```python
from build123d import *

# Parameters (mm, degrees)
SKETCH2_W               = 20
SKETCH2_H               = 10
BOSS_EXTRUDE1_DEPTH     = 132
SKETCH6_W               = 10
SKETCH6_H               = 3
BOSS_EXTRUDE2_DEPTH     = 10
FILLET2_R               = 10
CUT_EXTRUDE5_DEPTH      = 131.636901372
CUT_EXTRUDE5_DEPTH_BACK = 131.636901372
SKETCH19_R              = 1.5
SKETCH19_5_R            = 2.7
SKETCH19_5_R_2          = 1.5
CUT_EXTRUDE7_DEPTH      = 131.636901376
FILLET1_R               = 1
FILLET3_R               = 10
CUT_EXTRUDE8_DEPTH      = 131.636901391
CUT_EXTRUDE8_DEPTH_BACK = 131.636901391
SKETCH20_R              = 1.5
SKETCH20_3_R            = 2.7
SKETCH20_3_R_2          = 1.5
CUT_EXTRUDE9_DEPTH      = 131.636901391
SKETCH21_R              = 2.5
CUT_EXTRUDE10_DEPTH     = 10
FILLET4_R               = 15


# Some blends are built 0.0001 mm under size
with BuildPart() as part:
    # Sketch2 → Boss-Extrude1 (new body)
    with BuildSketch(Plane(origin=(0, 0, 0), x_dir=(1, 0, 0), z_dir=(0, 1, 0))):
        Rectangle(SKETCH2_W, SKETCH2_H)
    extrude(amount=BOSS_EXTRUDE1_DEPTH)

    # Sketch6 → Boss-Extrude2 (add)
    with BuildSketch(Plane(origin=(10, 0, 0), x_dir=(0, 0, -1), z_dir=(1, 0, 0))):
        with Locations((0, 1.5)):
            Rectangle(SKETCH6_W, SKETCH6_H)
    boss_extrude2 = extrude(amount=BOSS_EXTRUDE2_DEPTH)

    # Fillet2
    fillet2_edges = [part.edges().sort_by_distance(p)[0] for p in [
        (10, 3, 0),
    ]]
    fillet(fillet2_edges, radius=FILLET2_R - 0.0001)  # a hair under: the kernel refuses the full size

    # Sketch19 → Cut-Extrude5 (cut, two sides: drawn at the far end of the back side and taken through both)
    with BuildSketch(Plane(origin=(0, 3, 0), x_dir=(1, 0, 0), z_dir=(0, 1, 0)).offset(-CUT_EXTRUDE5_DEPTH_BACK)):
        with Locations(Location((15, 0, 0), (0, 0, 270))):
            Circle(SKETCH19_R)
    extrude(amount=CUT_EXTRUDE5_DEPTH + CUT_EXTRUDE5_DEPTH_BACK, mode=Mode.SUBTRACT)

    # Sketch19<5> → Cut-Extrude7 (cut, through all)
    with BuildSketch(Plane(origin=(0, 3, 0), x_dir=(1, 0, 0), z_dir=(0, 1, 0))):
        with Locations(Location((15, 0, 0), (0, 0, 90))):
            Circle(SKETCH19_5_R)
        with Locations(Location((15, 0, 0), (0, 0, 270))):
            Circle(SKETCH19_5_R_2, mode=Mode.SUBTRACT)
    extrude(amount=CUT_EXTRUDE7_DEPTH, mode=Mode.SUBTRACT)

    # Mirror16: Boss-Extrude2 across plane
    add(boss_extrude2.mirror(Plane(origin=(0, 0, 0), x_dir=(0, 0, 1), z_dir=(1, 0, 0))))

    # Fillet1
    fillet1_edges = [part.edges().sort_by_distance(p)[0] for p in [
        (20, 1.5, 5),
        (20, 1.5, -5),
        (-20, 1.5, 5),
        (-20, 1.5, -5),
    ]]
    fillet(fillet1_edges, radius=FILLET1_R)

    # Fillet3
    fillet3_edges = [part.edges().sort_by_distance(p)[0] for p in [
        (-10, 3, 0),
    ]]
    fillet(fillet3_edges, radius=FILLET3_R - 0.0001)  # a hair under: the kernel refuses the full size

    # Sketch20 → Cut-Extrude8 (cut, two sides: drawn at the far end of the back side and taken through both)
    with BuildSketch(Plane(origin=(0, 3, 0), x_dir=(1, 0, 0), z_dir=(0, 1, 0)).offset(-CUT_EXTRUDE8_DEPTH_BACK)):
        with Locations(Location((-14.5, 0, 0), (0, 0, 270))):
            Circle(SKETCH20_R)
    extrude(amount=CUT_EXTRUDE8_DEPTH + CUT_EXTRUDE8_DEPTH_BACK, mode=Mode.SUBTRACT)

    # Sketch20<3> → Cut-Extrude9 (cut, through all)
    with BuildSketch(Plane(origin=(0, 3, 0), x_dir=(1, 0, 0), z_dir=(0, 1, 0))):
        with Locations(Location((-14.5, 0, 0), (0, 0, 90))):
            Circle(SKETCH20_3_R)
        with Locations(Location((-14.5, 0, 0), (0, 0, 270))):
            Circle(SKETCH20_3_R_2, mode=Mode.SUBTRACT)
    extrude(amount=CUT_EXTRUDE9_DEPTH, mode=Mode.SUBTRACT)

    # Sketch21 → Cut-Extrude10 (cut)
    with BuildSketch(Plane.XY.offset(5)):
        with Locations((0, 125)):
            Circle(SKETCH21_R)
    extrude(amount=-CUT_EXTRUDE10_DEPTH, mode=Mode.SUBTRACT)

    # Fillet4
    # the kernel refuses this fillet: 15 mm, written as the material it takes off along each edge
    with BuildSketch(Plane(origin=(-10, 132, 42.5), x_dir=(0, -1, 0), z_dir=(0, 0, -1))) as fillet4_piece_1:
        with BuildLine():
            CenterArc((FILLET4_R, -FILLET4_R), FILLET4_R, 90, 90)
            Line((0, -FILLET4_R), (0, 0))
            Line((0, 0), (FILLET4_R, 0))
        make_face()
    extrude(amount=85, mode=Mode.SUBTRACT)
    with BuildSketch(Plane(origin=(10, 132, -42.5), x_dir=(-1, 0, 0), z_dir=(0, 0, 1))) as fillet4_piece_2:
        with BuildLine():
            CenterArc((FILLET4_R, FILLET4_R), FILLET4_R, 180, 90)
            Line((0, FILLET4_R), (0, 0))
            Line((0, 0), (FILLET4_R, 0))
        make_face()
    extrude(amount=85, mode=Mode.SUBTRACT)


solid = part.part
```
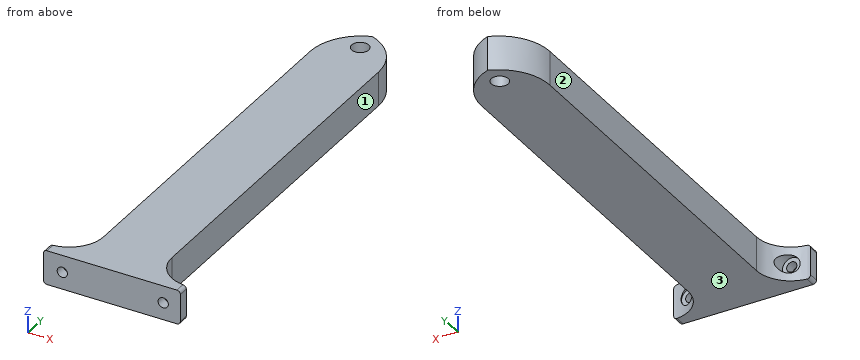
The listing builds one solid part. Answer for the finished solid, in the listing's coordinates (mm). Face numbers are marked on the shaded views. A direction names the side the tool comes from. Give positions to 0.01 mm unless a question says otherwise; leave off trailing zeros. Order: outer loops, then holes, each group sorted by start corner. A loop starts at its lowest first (then second) coordinate and runs counter-clockwise, first axis right, second up. Notation, with made-up numbers: (-3, -30) - (53, -30) arc R14 cw to (53, -20) - close; hole circle Ø5 at (-23.5, 74.25). An arc over 180 degrees is marked (long way). Answer in a Markdown table with one row per item. Add a question column.
Q1. The part is cut by section C-C (x = 15). Determine the outline of the cut face in (y, z), then the cut area to 3 significant figures.
Q2. Which of the six approach directions +Z, -Z, +X, -X, +Y, -Y give full straight-line access (tool end or side, diameter ignored) to the marked faces 1, 2 and 3?
Q3. Given P1, Ø4, axis at y = 118, z = 1, coming from the -X side; P2, Ø6, axis at x = -14.5, z = 0, coming from the +Y side; P3, Ø1.6, axis at x = 16, z = -1, coming from the +Y side, each flat-ended and moving along its own axis, determine where each tip first touches the part or whether it passes through.
Q4. The part is cut by section B-B (y = 125). Determine the outline of the cut face in (x, z).
Q5. Find the intervals of material crossed by line 1 along X through (y, z) = (2.2, 0); line 2 along Z through (x, y) = (15, 0.95); line 3 along X through (y, z) = (5.8, 0), in increasing order. Write a range as [from, to].
Q6. The part is cut by section D-D (y = 47). Determine the outline of the cut face in (x, z).
Q7. The part is cut by section A-A (z = 0). Give the number of separate pieces and of enclosed holes in the cut face, then the cut area to 3 significant figures.
Determined:
| question | item | result |
|---|---|---|
| 1 | outline | (0, -5) - (4.34, -5) - (4.34, -2.7) - (3, -2.7) - (3, -1.5) - (0, -1.5) - close; (0, 1.5) - (3, 1.5) - (3, 2.7) - (4.34, 2.7) - (4.34, 5) - (0, 5) - close |
| 1 | area | 27.2 mm² |
| 2 | face 1 | +Z, -Z, +X, +Y |
| 2 | face 2 | +Z, -Z, -X, +Y |
| 2 | face 3 | -Z, +X, -X, +Y, -Y |
| 3 | P1 | stops at x = -10 |
| 3 | P2 | stops at y = 7.73 |
| 3 | P3 | stops at y = 3 |
| 4 | outline | (-7.69, -5) - (-2.5, -5) - (-2.5, 5) - (-7.69, 5) - close; (2.5, -5) - (7.69, -5) - (7.69, 5) - (2.5, 5) - close |
| 5 | line 1 | x = [-20, -16], [-13, 13.5], [16.5, 20] |
| 5 | line 2 | z = [-5, -1.5], [1.5, 5] |
| 5 | line 3 | x = [-11.8, 12.3] |
| 6 | outline | (-10, -5) - (10, -5) - (10, 5) - (-10, 5) - close |
| 7 | separate pieces | 3 |
| 7 | enclosed holes | 1 |
| 7 | area | 2,590 mm² |
